```python
from build123d import *
from build123d.topology import SkipClean

# Parameters (mm, degrees)
SKETCH1_R                            = 7.5
SKETCH1_R_2                          = 2
BOSS_EXTRUDE1_DEPTH                  = 10
BOSS_EXTRUDE1_2_DEPTH                = 10
BOSS_EXTRUDE2_REACH                  = 159.995
BOSS_EXTRUDE2_END_RADIUS             = 7.5
SKETCH2_R                            = 5
BOSS_EXTRUDE2_DIRECTION_2_REACH      = 159.995
BOSS_EXTRUDE2_DIRECTION_2_END_RADIUS = 7.5


with BuildPart() as part:
    # Sketch1 → Boss-Extrude1 (new body)
    with BuildSketch(Plane(origin=(0, 0, 0), x_dir=(1, 0, 0), z_dir=(0, 1, 0))):
        with Locations(Location((0, 0, 0), (0, 0, 270))):
            Circle(SKETCH1_R)
        with Locations(Location((0, 0, 0), (0, 0, 270))):
            Circle(SKETCH1_R_2, mode=Mode.SUBTRACT)
    extrude(amount=BOSS_EXTRUDE1_DEPTH)



with BuildPart() as body_2:
    # Sketch1 → Boss-Extrude1 2 (new body)
    with BuildSketch(Plane(origin=(0, 0, 0), x_dir=(1, 0, 0), z_dir=(0, 1, 0))):
        with Locations(Location((300, 0, 0), (0, 0, 270))):
            Circle(SKETCH1_R)
        with Locations(Location((300, 0, 0), (0, 0, 270))):
            Circle(SKETCH1_R_2, mode=Mode.SUBTRACT)
    extrude(amount=BOSS_EXTRUDE1_2_DEPTH)


with BuildPart() as part_1:
    with SkipClean():  # the faces are left unmerged after this step: merging them gives an invalid solid
        add(part.part)

        add(body_2.part)  # Boss-Extrude2 merges body 2
        # Boss-Extrude2: up to this cylinder (the profile starts outside it)
        boss_extrude2_end = Plane(origin=(300, 5, 0), z_dir=(0, -1, 0)) * Cylinder(BOSS_EXTRUDE2_END_RADIUS, 335.99, mode=Mode.PRIVATE)
        # Sketch2 → Boss-Extrude2 (add, up to the surface)
        with BuildSketch(Plane(origin=(150, 0, 0), x_dir=(0, 0, -1), z_dir=(1, 0, 0)), mode=Mode.PRIVATE) as boss_extrude2_sk1:
            with Locations(Location((0, 5, 0), (0, 0, 90))):
                Circle(SKETCH2_R)
        boss_extrude2_tool1 = extrude(boss_extrude2_sk1.sketch, amount=BOSS_EXTRUDE2_REACH, mode=Mode.PRIVATE) - boss_extrude2_end
        add(boss_extrude2_tool1.solids().sort_by_distance((150, 5, 0))[0])

    # Boss-Extrude2 direction 2: up to this cylinder (the profile starts outside it)
    boss_extrude2_direction_2_end = Plane(origin=(0, 5, 0), z_dir=(0, -1, 0)) * Cylinder(BOSS_EXTRUDE2_DIRECTION_2_END_RADIUS, 335.99, mode=Mode.PRIVATE)
    # Sketch2 → Boss-Extrude2 direction 2 (add, up to the surface)
    with BuildSketch(Plane(origin=(150, 0, 0), x_dir=(0, 0, -1), z_dir=(1, 0, 0)), mode=Mode.PRIVATE) as boss_extrude2_direction_2_sk1:
        with Locations(Location((0, 5, 0), (0, 0, 90))):
            Circle(SKETCH2_R)
    boss_extrude2_direction_2_tool1 = extrude(boss_extrude2_direction_2_sk1.sketch, amount=-BOSS_EXTRUDE2_DIRECTION_2_REACH, mode=Mode.PRIVATE) - boss_extrude2_direction_2_end
    add(boss_extrude2_direction_2_tool1.solids().sort_by_distance((150, 5, 0))[0])


solid = part_1.part
```
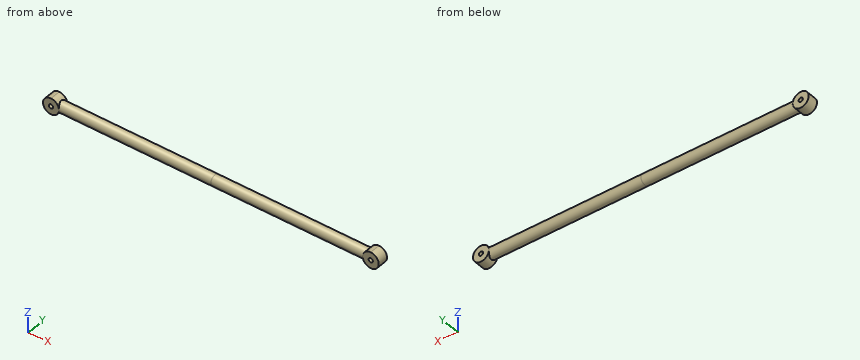
Design review of the part built by this model. Coordinates are the model's own, in mm. Coordinates: 2 decimals unless noted, no trailing zeros. Loops run counter-clockwise (first coordinate to the right, second up) from the corner with the lowest first, then second, coordinate; pieces in that order, holes last. Notation, with made-up numbers: (15, 35.5) - (39, 35.5) arc R22 cw to (39, 51.5) - close; hole circle Ø8 at (72, 72.5). An arc over 180 degrees is marked (long way). Use CSV: the item, a comma, the result in double quotes. Start each with the question number.
1) Consider section A-A on y = 5. Write out the cut boundary in (x, z).
2) Consider section B-B on x = 220. Write out the cut boundary in (y, z).
3) Wall thickness on L1, parallel to X at y = 5.25, z = 0; L2, parallel to X at y = 2.25, z = 0.5; L3, parallel to Z at x = 300, y = 7: over which ranges is each line inside the solid? List them lowest first. Write a range as from..to.
4) For pin 1 Ø1 at (x, y) = (206.5, 5) entering from -Z; pin 2 Ø3 at (x, z) = (66, 0.5) entering from +Y; pin 3 Ø4 at (x, y) = (130.5, 1) entering from -Z; pin 4 Ø3 at (y, z) = (4.5, 5.5) entering from +X, all flat-tipped, find the tip position at first contact; note any pin that passes through.
Geometry says:
1,outline,"(5.59, -5) - (294.41, -5) arc R7.5 ccw (long way) to (294.41, 5) - (5.59, 5) arc R7.5 ccw (long way) to start; hole circle Ø4 at (0, 0); hole circle Ø4 at (300, 0)"
2,outline,"circle Ø10 at (5, 0)"
3,L1,"-7.5..-2, 2..298, 302..307.5"
3,L2,"-7.48..-1.94, 1.94..298.06, 301.94..307.48"
3,L3,"-7.5..-2, 2..7.5"
4,pin 1,"z = -5"
4,pin 2,"y = 10"
4,pin 3,"z = -4.58"
4,pin 4,"x = 306.34"
